from build123d import *

# Parameters (mm, degrees)
ESQUISSE1_W                  = 6.94
ESQUISSE1_H                  = 12.9
BOSS_EXTRU_1_DEPTH           = 9.06
ESQUISSE2_R                  = 2.85
BOSS_EXTRU_2_DEPTH           = 8.7
ESQUISSE3_R                  = 2
ENL_V_MAT_EXTRU_1_DEPTH      = 8.7
ENL_V_MAT_EXTRU_2_DEPTH      = 2.5
ENL_V_MAT_EXTRU_2_DEPTH_BACK = 2.5
ENL_V_MAT_EXTRU_2_START      = -3.45
ESQUISSE4_R                  = 0.5
CHANFREIN1_SIZE              = 0.25
CHANFREIN1_SIZE2             = 2.378591114
ESQUISSE5_W                  = 2.16
ESQUISSE5_H                  = 0.8
BOSS_EXTRU_3_DEPTH           = 4
CONG_1_R                     = 0.3
ESQUISSE6_W                  = 1.1
ESQUISSE6_H                  = 1.9
ENL_V_MAT_EXTRU_3_DEPTH      = 23.371213646


with BuildPart() as part:
    # Esquisse1 → Boss.-Extru.1 (new body)
    with BuildSketch(Plane(origin=(0, 0, 0), x_dir=(1, 0, 0), z_dir=(0, 1, 0))):
        with Locations((3.47, 6.45)):
            Rectangle(ESQUISSE1_W, ESQUISSE1_H)
    extrude(amount=BOSS_EXTRU_1_DEPTH)

    # Esquisse2 → Boss.-Extru.2 (add)
    with BuildSketch(Plane(origin=(0, 9.06, 0), x_dir=(1, 0, 0), z_dir=(0, 1, 0))):
        with Locations(Location((3.47, 6.45, 0), (0, 0, 90))):
            Circle(ESQUISSE2_R)
    extrude(amount=BOSS_EXTRU_2_DEPTH)

    # Esquisse3 → Enlèv. mat.-Extru.1 (cut)
    with BuildSketch(Plane(origin=(0, 17.76, 0), x_dir=(1, 0, 0), z_dir=(0, 1, 0))):
        with Locations(Location((3.47, 6.45, 0), (0, 0, 270))):
            Circle(ESQUISSE3_R)
    extrude(amount=-ENL_V_MAT_EXTRU_1_DEPTH, mode=Mode.SUBTRACT)

    # Esquisse4 → Enlèv. mat.-Extru.2 (cut, two sides: drawn at the far end of the back side and taken through both)
    with BuildSketch(Plane.ZY.offset(ENL_V_MAT_EXTRU_2_START - ENL_V_MAT_EXTRU_2_DEPTH_BACK)):
        with Locations(Location((-6.453279692, 14.76, 0), (0, 0, 180))):
            Circle(ESQUISSE4_R)
    extrude(amount=ENL_V_MAT_EXTRU_2_DEPTH + ENL_V_MAT_EXTRU_2_DEPTH_BACK, mode=Mode.SUBTRACT)

    # Chanfrein1
    chanfrein1_edges = [part.edges().sort_by_distance(p)[0] for p in [
        (3.47, 17.76, -8.45),
    ]]
    chanfrein1_side = [part.faces().sort_by_distance(p)[0] for p in [
        (3.47, 17.76, -3.680610173),
    ]]
    chamfer(chanfrein1_edges, length=CHANFREIN1_SIZE, length2=CHANFREIN1_SIZE2, reference=chanfrein1_side[0])

    # Esquisse5 → Boss.-Extru.3 (add)
    with BuildSketch(Plane.XZ):
        with Locations((3.47, -1.6)):
            Rectangle(ESQUISSE5_W, ESQUISSE5_H)
        with Locations((3.47, -11.3)):
            Rectangle(ESQUISSE5_W, ESQUISSE5_H)
        with Locations((3.47, -6.45)):
            Rectangle(ESQUISSE5_W, ESQUISSE5_H)
    extrude(amount=BOSS_EXTRU_3_DEPTH)

    # Congé1
    cong_1_edges = [part.edges().sort_by_distance(p)[0] for p in [
        (2.39, -4, -1.6),
        (4.55, -4, -1.6),
        (4.55, -4, -11.3),
        (2.39, -4, -11.3),
        (2.39, -4, -6.45),
        (4.55, -4, -6.45),
    ]]
    fillet(cong_1_edges, radius=CONG_1_R)

    # Esquisse6 → Enlèv. mat.-Extru.3 (cut, through all)
    with BuildSketch(Plane(origin=(0, 0, -11.7), x_dir=(-1, 0, 0), z_dir=(0, 0, -1))):
        with Locations((-3.470290463, -2.41)):
            Rectangle(ESQUISSE6_W, ESQUISSE6_H)
    extrude(amount=-ENL_V_MAT_EXTRU_3_DEPTH, mode=Mode.SUBTRACT)


solid = part.part
Here's how the part is built. I have some questions about the finished solid (model axes, mm). A direction names the side the tool comes from. Round coordinates to 2 decimals unless told otherwise and drop trailing zeros. Order: outer loops, then holes, each group sorted by start corner. A loop starts at its lowest first (then second) coordinate and runs counter-clockwise, first axis right, second up. Notation, with made-up numbers: (12, 71.5) -> (48, 71.5) arc R27 ccw to (48, 105.5) -> close; hole circle Ø9 at (-23, 3). An arc over 180 degrees is marked (long way). Use CSV: the item, a comma, the result in double quotes.
1. I need wall thicknesses on line 1 along X through (y, z) = (13, -6.45); line 2 along Y through (x, z) = (3, -10.25); line 3 along X through (y, z) = (-1.75, -6.75). Which ranges of each line are inside material? Lowest first, please.
Recorded:
line 1,"x = 0.62 to 1.47, 5.47 to 6.32"
line 2,"y = 0 to 9.06"
line 3,"x = 2.39 to 2.92, 4.02 to 4.55"
2. I want a section at D-D on z = -9. List the corners of the cut face in (x, y) for me, and give its area (3 significant figures).
Recorded:
outline,"(0, 0) -> (6.94, 0) -> (6.94, 9.06) -> (4.74, 9.06) -> (4.74, 17.76) -> (2.2, 17.76) -> (2.2, 9.06) -> (0, 9.06) -> close"
area,"85.0 mm2"
3. I want a section at C-C on x = 3.47. Give the number of separate pieces and of enclosed holes in the cut face, and give its area (3 significant figures).
Recorded:
separate pieces,"4"
enclosed holes,"0"
area,"136 mm2"
4. Which directions (+Z, -Z, +X, -X, +Y, -Y) give clear straight access to the entire face, cutting with the end or side of a thin tool? Please do faces 5 (the face through (3.5, -1.46, -6.5)), 6 (the face through (4.55, -1.8, -6.5)), 7 (the face through (3, 9.06, -6)), 8 (the face through (3, -1, -6.05)), 9 (the face through (0.95, 14.8, -6.4)).
Recorded:
face 5,"+Z, -Z"
face 6,"+Z, -Z, +X, -Y"
face 7,"+Y"
face 8,"+X, -X, -Y"
face 9,"none"
5. I'm going to push flat-ended pins straight in: P1, Ø2.5, axis at x = 3.5, y = -1.5, coming from the +Z side; P2, Ø1.7, axis at x = 3.5, y = -1.5, coming from the -Z side; P3, Ø0.6, axis at y = -2.5, z = -1.5, coming from the -X side; P4, Ø1.5, axis at x = 3, z = -8.5, coming from the +Y side. Where does each tip first touch, or does it pass through?
Recorded:
P1,"stops at z = -1.2"
P2,"stops at z = -11.7"
P3,"stops at x = 2.39"
P4,"stops at y = 17.76"
6. I want a section at A-A on z = -11.25. List the corners of the cut face in (x, y) for me.
Recorded:
outline,"(0, 0) -> (2.39, 0) -> (2.39, -3.7) arc R0.3 ccw to (2.69, -4) -> (4.25, -4) arc R0.3 ccw to (4.55, -3.7) -> (4.55, 0) -> (6.94, 0) -> (6.94, 9.06) -> (0, 9.06) -> close; hole (2.92, -3.36) -> (4.02, -3.36) -> (4.02, -1.46) -> (2.92, -1.46) -> close"
7. I want a section at B-B on y = 14.76. List the corners of the cut face in (x, z) for me.
Recorded:
outline,"circle Ø5.7 at (3.47, -6.45); hole (0.95, -6.95) -> (1.53, -6.95) arc R2 ccw to (5.41, -6.95) -> (5.95, -6.95) -> (5.95, -5.95) -> (5.41, -5.95) arc R2 ccw to (1.53, -5.95) -> (0.95, -5.95) -> close"
8. Thinking about a two-plate mould opening in X: for faces 1 (the face through (3, -1, -11.7)), 2 (the face through (5.682, 14.738, -5.954)), 3 (the face through (4.02, -2.4, -1.6)), 4 (the face through (2.39, -1.8, -11.3)), which applies, pulls with the +X half, pulls with the -X half, needs draft (parallel to the pull), parting line crosses it, or undercut?
Recorded:
face 1,"needs draft"
face 2,"undercut"
face 3,"undercut"
face 4,"pulls with the -X half"
